Answer from the drawing. Dimensions are ordinates in mm from the lowest x, y and z of the part. A direction names the side the tool comes from. Coordinates: 2 decimals unless noted, no trailing zeros. Loops run counter-clockwise (first coordinate to the right, second up) from the corner with the lowest first, then second, coordinate; pieces in that order, holes last.
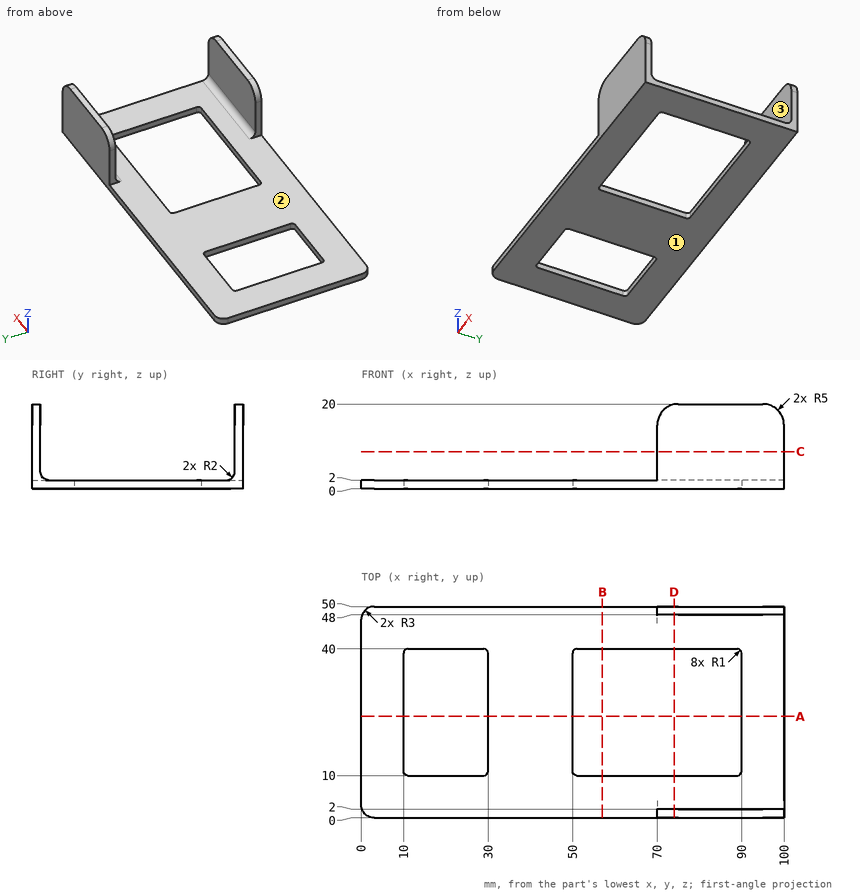
Item 1: Given pin 1 (1.5 mm diameter, centred on y = 33, z = 4.5, fed in from -X); pin 2 (3 mm diameter, centred on x = 10.5, y = 21, fed in from +Z); pin 3 (4.5 mm diameter, centred on y = 48.5, z = 7.5, fed in from -X), each flat-ended and moving along its own axis, determine where each tip first touches the part or whether it passes through.
Numbers:
pin 1: passes through
pin 2: stops at z = 2
pin 3: stops at x = 70
Item 2: Which of the six approach directions +Z, -Z, +X, -X, +Y, -Y give full straight-line access (tool end or side, diameter ignored) to the marked faces 1, 2 and 3?
Numbers:
face 1: -Z, +X, -X, +Y, -Y
face 2: +Z, -X
face 3: +Z, +X, -X
Item 3: A cutting plane is placed at B-B on x = 57. Determine the outline of the cut face in (y, z).
Numbers:
outline: (0, 0) - (10, 0) - (10, 2) - (0, 2) - close; (40, 0) - (50, 0) - (50, 2) - (40, 2) - close
Item 4: A cutting plane is placed at D-D on x = 74. Determine the outline of the cut face in (y, z).
Numbers:
outline: (0, 0) - (10, 0) - (10, 2) - (4, 2) arc R2 cw to (2, 4) - (2, 19.9) - (0, 19.9) - close; (40, 0) - (50, 0) - (50, 19.9) - (48, 19.9) - (48, 4) arc R2 cw to (46, 2) - (40, 2) - close
Item 5: Find the intervals of material crossed by line 1 along Y through (x, z) = (96, 5); line 2 along Z through (x, y) = (88, 44.5), in increasing order.
Numbers:
line 1: y = 0 to 2, 48 to 50
line 2: z = 0 to 2
Item 6: A cutting plane is placed at C-C on z = 8.75. Determine the outline of the cut face in (x, y), then the cut area to 3 significant figures.
Numbers:
outline: (70, 0) - (100, 0) - (100, 2) - (70, 2) - close; (70, 48) - (100, 48) - (100, 50) - (70, 50) - close
area: 120 mm2
Item 7: A cutting plane is placed at A-A on y = 24. Determine the outline of the cut face in (x, z).
Numbers:
outline: (0, 0) - (10, 0) - (10, 2) - (0, 2) - close; (30, 0) - (50, 0) - (50, 2) - (30, 2) - close; (90, 0) - (100, 0) - (100, 2) - (90, 2) - close
